```python
from build123d import *

# Parameters (mm, degrees)
SKETCH1_W                  = 277.368
SKETCH1_H                  = 57.15
BOSS_EXTRUDE1_DEPTH        = 3.175
SKETCH2_W                  = 277.368
SKETCH2_H                  = 25.4
BOSS_EXTRUDE2_DEPTH        = 3.175
SKETCH3_W                  = 277.368
SKETCH3_H                  = 25.4
BOSS_EXTRUDE3_DEPTH        = 3.175
BOSS_EXTRUDE4_DEPTH        = 2.54
BOSS_EXTRUDE5_DEPTH        = 2.54
BOSS_EXTRUDE6_DEPTH        = 2.54
BOSS_EXTRUDE7_DEPTH        = 2.54
BOSS_EXTRUDE8_DEPTH        = 2.54
BOSS_EXTRUDE9_DEPTH        = 2.54
F_10_CLEARANCE_HOLE1_D     = 5.1054
F_10_CLEARANCE_HOLE1_DEPTH = 3.175
F_10_CLEARANCE_HOLE2_D     = 5.1054
F_10_CLEARANCE_HOLE2_DEPTH = 3.175
F_10_CLEARANCE_HOLE3_D     = 4.9784
F_10_CLEARANCE_HOLE3_DEPTH = 3.175
F_10_CLEARANCE_HOLE4_D     = 4.9784
SKETCH22_R                 = 3.770312501
SKETCH22_R_2               = 4.062065624
BOSS_EXTRUDE10_DEPTH       = 3.175


with BuildPart() as part:
    # Sketch1 → Boss-Extrude1 (new body)
    with BuildSketch(Plane.XY):
        with Locations((138.684, 28.575)):
            Rectangle(SKETCH1_W, SKETCH1_H)
        with BuildLine():
            Line((30.185295474, 13.081), (12.359704526, 43.955829198))
            ThreePointArc((12.359704526, 43.955829198), (12.359704526, 46.495829198), (14.559409051, 47.765829198))
            Line((14.559409051, 47.765829198), (50.210590949, 47.765829198))
            ThreePointArc((50.210590949, 47.765829198), (52.410295474, 46.495829198), (52.410295474, 43.955829198))
            Line((52.410295474, 43.955829198), (34.584704526, 13.081))
            ThreePointArc((34.584704526, 13.081), (32.385, 11.811), (30.185295474, 13.081))
        make_face(mode=Mode.SUBTRACT)
        with BuildLine():
            Line((49.484409051, 9.271), (85.135590949, 9.271))
            ThreePointArc((85.135590949, 9.271), (87.335295474, 10.541), (87.335295474, 13.081))
            Line((87.335295474, 13.081), (69.509704526, 43.955829198))
            ThreePointArc((69.509704526, 43.955829198), (67.31, 45.225829198), (65.110295474, 43.955829198))
            Line((65.110295474, 43.955829198), (47.284704526, 13.081))
            ThreePointArc((47.284704526, 13.081), (47.284704526, 10.541), (49.484409051, 9.271))
        make_face(mode=Mode.SUBTRACT)
        with BuildLine():
            Line((100.035295474, 13.081), (82.209704526, 43.955829198))
            ThreePointArc((82.209704526, 43.955829198), (82.209704526, 46.495829198), (84.409409051, 47.765829198))
            Line((84.409409051, 47.765829198), (120.060590949, 47.765829198))
            ThreePointArc((120.060590949, 47.765829198), (122.260295474, 46.495829198), (122.260295474, 43.955829198))
            Line((122.260295474, 43.955829198), (104.434704526, 13.081))
            ThreePointArc((104.434704526, 13.081), (102.235, 11.811), (100.035295474, 13.081))
        make_face(mode=Mode.SUBTRACT)
        with BuildLine():
            Line((119.334409051, 9.271), (154.985590949, 9.271))
            ThreePointArc((154.985590949, 9.271), (157.185295474, 10.541), (157.185295474, 13.081))
            Line((157.185295474, 13.081), (139.359704526, 43.955829198))
            ThreePointArc((139.359704526, 43.955829198), (137.16, 45.225829198), (134.960295474, 43.955829198))
            Line((134.960295474, 43.955829198), (117.134704526, 13.081))
            ThreePointArc((117.134704526, 13.081), (117.134704526, 10.541), (119.334409051, 9.271))
        make_face(mode=Mode.SUBTRACT)
        with BuildLine():
            Line((169.885295474, 13.081), (152.059704526, 43.955829198))
            ThreePointArc((152.059704526, 43.955829198), (152.059704526, 46.495829198), (154.259409051, 47.765829198))
            Line((154.259409051, 47.765829198), (189.910590949, 47.765829198))
            ThreePointArc((189.910590949, 47.765829198), (192.110295474, 46.495829198), (192.110295474, 43.955829198))
            Line((192.110295474, 43.955829198), (174.284704526, 13.081))
            ThreePointArc((174.284704526, 13.081), (172.085, 11.811), (169.885295474, 13.081))
        make_face(mode=Mode.SUBTRACT)
        with BuildLine():
            Line((189.184409051, 9.271), (224.835590949, 9.271))
            ThreePointArc((224.835590949, 9.271), (227.035295474, 10.541), (227.035295474, 13.081))
            Line((227.035295474, 13.081), (209.209704526, 43.955829198))
            ThreePointArc((209.209704526, 43.955829198), (207.01, 45.225829198), (204.810295474, 43.955829198))
            Line((204.810295474, 43.955829198), (186.984704526, 13.081))
            ThreePointArc((186.984704526, 13.081), (186.984704526, 10.541), (189.184409051, 9.271))
        make_face(mode=Mode.SUBTRACT)
        with BuildLine():
            Line((239.735295474, 13.081), (221.909704526, 43.955829198))
            ThreePointArc((221.909704526, 43.955829198), (221.909704526, 46.495829198), (224.109409051, 47.765829198))
            Line((224.109409051, 47.765829198), (259.760590949, 47.765829198))
            ThreePointArc((259.760590949, 47.765829198), (261.960295474, 46.495829198), (261.960295474, 43.955829198))
            Line((261.960295474, 43.955829198), (244.134704526, 13.081))
            ThreePointArc((244.134704526, 13.081), (241.935, 11.811), (239.735295474, 13.081))
        make_face(mode=Mode.SUBTRACT)
    extrude(amount=BOSS_EXTRUDE1_DEPTH)

    # Sketch2 → Boss-Extrude2 (add)
    with BuildSketch(Plane(origin=(0, 57.15, 0), x_dir=(1, 0, 0), z_dir=(0, 1, 0))):
        with Locations((138.684, -12.7)):
            Rectangle(SKETCH2_W, SKETCH2_H)
    extrude(amount=-BOSS_EXTRUDE2_DEPTH)

    # Sketch3 → Boss-Extrude3 (add)
    with BuildSketch(Plane.XZ):
        with Locations((138.684, 12.7)):
            Rectangle(SKETCH3_W, SKETCH3_H)
    extrude(amount=-BOSS_EXTRUDE3_DEPTH)

    # Sketch5 → Boss-Extrude4 (add)
    with BuildSketch(Plane.YZ.offset(43.18)):
        Polygon((3.175, 3.175), (3.175, 25.4), (25.4, 3.175), align=None)
    extrude(amount=BOSS_EXTRUDE4_DEPTH)

    # Sketch6 → Boss-Extrude5 (add)
    with BuildSketch(Plane.YZ.offset(113.03)):
        Polygon((3.175, 25.4), (3.175, 3.175), (25.4, 3.175), align=None)
    extrude(amount=BOSS_EXTRUDE5_DEPTH)

    # Sketch7 → Boss-Extrude6 (add)
    with BuildSketch(Plane.YZ.offset(182.88)):
        Polygon((3.175, 25.4), (3.175, 3.175), (25.4, 3.175), align=None)
    extrude(amount=BOSS_EXTRUDE6_DEPTH)

    # Sketch8 → Boss-Extrude7 (add)
    with BuildSketch(Plane(origin=(76.708, 0, 0), x_dir=(0, -1, 0), z_dir=(-1, 0, 0))):
        Polygon((-53.975, 3.175), (-53.975, 25.4), (-31.75, 3.175), align=None)
    extrude(amount=-BOSS_EXTRUDE7_DEPTH)

    # Sketch9 → Boss-Extrude8 (add)
    with BuildSketch(Plane(origin=(146.558, 0, 0), x_dir=(0, -1, 0), z_dir=(-1, 0, 0))):
        Polygon((-53.975, 25.4), (-53.975, 3.175), (-31.75, 3.175), align=None)
    extrude(amount=-BOSS_EXTRUDE8_DEPTH)

    # Sketch10 → Boss-Extrude9 (add)
    with BuildSketch(Plane(origin=(216.408, 0, 0), x_dir=(0, -1, 0), z_dir=(-1, 0, 0))):
        Polygon((-53.975, 25.4), (-53.975, 3.175), (-31.75, 3.175), align=None)
    extrude(amount=-BOSS_EXTRUDE9_DEPTH)

    # #10 Clearance Hole1
    with Locations(Plane(origin=(0, 3.175, 0), x_dir=(1, 0, 0), z_dir=(0, 1, 0))):
        with Locations((209.299668917, -15.125), (234.699668917, -15.125)):
            Hole(F_10_CLEARANCE_HOLE1_D / 2, depth=F_10_CLEARANCE_HOLE1_DEPTH)

    # #10 Clearance Hole2
    with Locations(Plane(origin=(0, 3.175, 0), x_dir=(1, 0, 0), z_dir=(0, 1, 0))):
        with Locations((264.668, -12.7)):
            Hole(F_10_CLEARANCE_HOLE2_D / 2, depth=F_10_CLEARANCE_HOLE2_DEPTH)

    # #10 Clearance Hole3
    with Locations(Plane(origin=(0, 3.175, 0), x_dir=(1, 0, 0), z_dir=(0, 1, 0))):
        with Locations((138.684, -12.7), (12.7, -12.7)):
            Hole(F_10_CLEARANCE_HOLE3_D / 2, depth=F_10_CLEARANCE_HOLE3_DEPTH)

    # #10 Clearance Hole4 (through all)
    with Locations(Plane(origin=(0, 53.975, 0), x_dir=(-1, 0, 0), z_dir=(0, -1, 0))):
        with Locations((-138.684, -12.7), (-264.668, -12.7), (-12.7, -12.7)):
            Hole(F_10_CLEARANCE_HOLE4_D / 2)

    # Sketch22 → Boss-Extrude10 (add)
    with BuildSketch(Plane.XZ.offset(-53.975)):
        with Locations((234.69966892, 15.125)):
            Circle(SKETCH22_R)
        with Locations((209.29966892, 15.125)):
            Circle(SKETCH22_R_2)
    extrude(amount=-BOSS_EXTRUDE10_DEPTH)


solid = part.part
```
For this review, take the finished solid that the model builds, in its own axes (mm). A direction names the side the tool comes from. Round coordinates to 2 decimals unless told otherwise and drop trailing zeros. Put each result on its own line as item: value.
Q1. We need section B-B (y = 36.5). Count the separate pieces of the cut face and the enclosed holes in it, and give its area (3 significant figures).
Solved:
separate pieces: 8
enclosed holes: 0
area: 394 mm2
Q2. Machinability: for faces 1 (the face through (231, 3.175, 14)), 2 (the face through (113.47, 28.73, 1.57)), 3 (the face through (77.96, 43.018, 14.443)), which of the approach directions +Z, -Z, +X, -X, +Y, -Y give a long, thin tool a straight path to every point of the face, cutting with its end or side? Answer none if there is none.
Solved:
face 1: +Z, +X
face 2: +Z, -Z
face 3: +Z, +X, -X
Q3. Wall thickness on probe 1 along X at (y, z) = (23, 5.5); probe 2 along Y at (x, z) = (177, 14.75) (3 decimals); probe 3 along X at (y, z) = (44, 10.5): over which ranges is each line inside the solid? List them lowest first.
Solved:
probe 1: x = 43.18 to 45.72, 113.03 to 115.57, 182.88 to 185.42
probe 2: y = 0 to 3.175, 53.975 to 57.15
probe 3: x = 76.71 to 79.25, 146.56 to 149.1, 216.41 to 218.95
Q4. Mouldability with a two-part tool opening along Y and no side actions: class faces 4 (the face through (137, 0, 15)), 5 (the face through (218.948, 48, 10)), 6 (the face through (136.849, 55.585, 11.018)) as released by +Y, released by -Y, zero draft, split by the parting line, or undercut.
Solved:
face 4: released by -Y
face 5: undercut
face 6: zero draft
Q5. Insertion check: pin 1 Ø11 at (y, z) = (46.5, 9.5) entering from -X; pin 2 Ø11 at (y, z) = (16, 11.5) entering from -X; pin 3 Ø11 at (y, z) = (38.5, 18) entering from +X; pin 4 Ø1.5 at (x, y) = (192.5, 39.5) entering from +Z (3 decimals). Each pin has a flat end and moves straight along its axis. Give the tip position at first contact, or say it passes through.
Solved:
pin 1: stops at x = 76.71
pin 2: stops at x = 43.18
pin 3: passes through
pin 4: stops at z = 3.175
